For this review, use the dimensioned drawing (mm, ordinates from the lowest corner) and the shaded views. Round coordinates to 2 decimals unless told otherwise and drop trailing zeros. Loops run counter-clockwise (first coordinate to the right, second up) from the corner with the lowest first, then second, coordinate; pieces in that order, holes last. Notation, with made-up numbers: (62, 60.5) - (101, 60.5) arc R10 ccw to (101, 65.5) - close; hole circle Ø4 at (-29.5, 10). An arc over 180 degrees is marked (long way). Use one line per item in the form item = value. Start each with the question number.
(1) We need section C-C, the plane x = 85. Write out the cut boundary in (y, z), then the cut area to 3 significant figures.
(2) We need section D-D, the plane x = 50. Write out the cut boundary in (y, z), then the cut area to 3 significant figures.
(3) We need section B-B, the plane z = 2.3. Write out the cut boundary in (x, y) (3 decimals).
(4) We need section A-A, the plane y = 25. Write out the cut boundary in (x, z), then the cut area to 3 significant figures.
(5) For pin 1 (1 mm diameter, centred on y = 38.5, z = 0.5, fed in from -X); pin 2 (1.5 mm diameter, centred on x = 1.5, z = 1.5, fed in from -Y) (3 decimals), all flat-tipped, find the tip position at first contact; note any pin that passes through.
(6) Wall thickness on probe 1 along Y at (x, z) = (85, 1); probe 2 along Y at (x, z) = (50, 1.4); probe 3 along Y at (x, z) = (54, 2.6): over which ranges is each line inside the solid? List them lowest first. Write a range as [from, to].
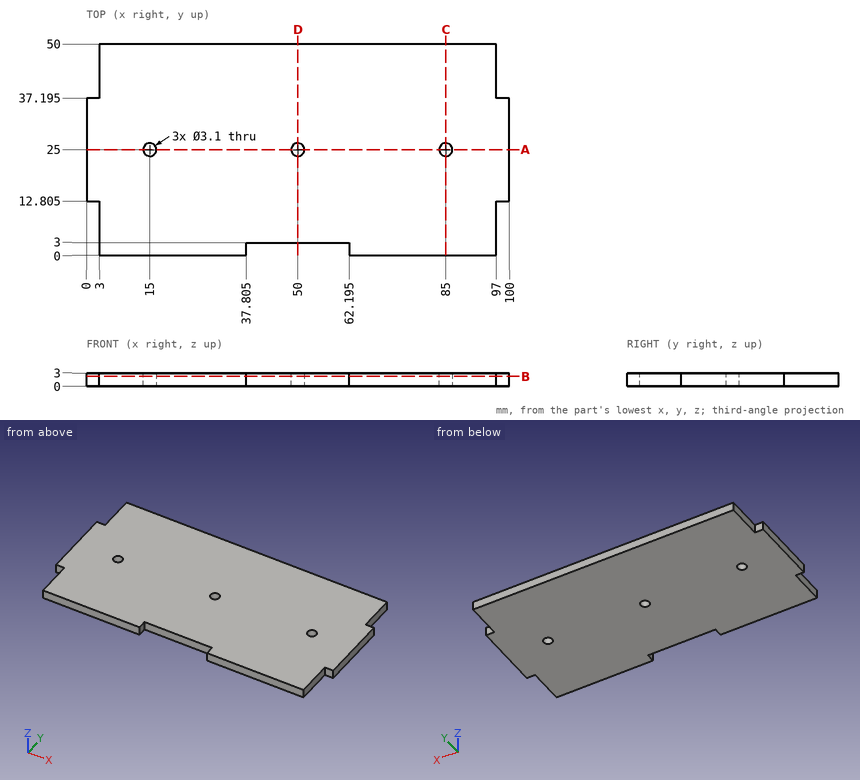
Data:
q1.outline = (0, 0) - (23.45, 0) - (23.45, 3) - (0, 3) - close; (26.55, 0) - (50, 0) - (50, 3) - (26.55, 3) - close
q1.area = 141 mm^2
q2.outline = (3, 0) - (23.45, 0) - (23.45, 3) - (3, 3) - close; (26.55, 0) - (50, 0) - (50, 3) - (26.55, 3) - close
q2.area = 132 mm^2
q3.outline = (0, 12.805) - (3, 12.805) - (3, 0) - (37.805, 0) - (37.805, 3) - (62.195, 3) - (62.195, 0) - (97, 0) - (97, 12.805) - (100, 12.805) - (100, 37.195) - (97, 37.195) - (97, 50) - (3, 50) - (3, 37.195) - (0, 37.195) - close; hole circle Ø3.1 at (15, 25); hole circle Ø3.1 at (50, 25); hole circle Ø3.1 at (85, 25)
q4.outline = (0, 0) - (13.45, 0) - (13.45, 3) - (0, 3) - close; (16.55, 0) - (48.45, 0) - (48.45, 3) - (16.55, 3) - close; (51.55, 0) - (83.45, 0) - (83.45, 3) - (51.55, 3) - close; (86.55, 0) - (100, 0) - (100, 3) - (86.55, 3) - close
q4.area = 272 mm^2
q5.pin_1 = 3
q5.pin_2 = 12.805
q6.probe_1 = [0, 23.45], [26.55, 50]
q6.probe_2 = [3, 23.45], [26.55, 50]
q6.probe_3 = [3, 50]
